Input: part model. Units: mm. Frame: model coordinates. A direction names the side the tool comes from. Round coordinates to 2 decimals unless told otherwise and drop trailing zeros. Loops run counter-clockwise (first coordinate to the right, second up) from the corner with the lowest first, then second, coordinate; pieces in that order, holes last. Notation, with made-up numbers: (85, 37.5) - (129, 37.5) arc R16 ccw to (129, 67.5) - close; hole circle Ø6 at (47.5, 63.5). An arc over 180 degrees is marked (long way). Write each question's results on one line, items separated by ' | '.
from build123d import *

# Parameters (mm, degrees)
EXTRUDE_1_DEPTH     = 15
SKETCH_2_W          = 4
SKETCH_2_H          = 60
EXTRUDE_2_DEPTH     = 10
SKETCH_3_R          = 1.6
CUT_EXTRUDE_1_DEPTH = 6


with BuildPart() as part:
    # ｽｹｯﾁ1 → ﾎﾞｽ - 押し出し1 (new body)
    with BuildSketch(Plane.XY):
        Polygon((-37.26940162, 16.179775281), (-33.26940162, 16.179775281), (-33.26940162, -39.820224719), (-3.26940162, -39.820224719), (-3.26940162, -43.820224719), (-37.26940162, -43.820224719), align=None)
    extrude(amount=EXTRUDE_1_DEPTH)

    # ｽｹｯﾁ2 → ﾎﾞｽ - 押し出し2 (add)
    with BuildSketch(Plane.ZY.offset(37.26940162)):
        with Locations((13, -13.820224719)):
            Rectangle(SKETCH_2_W, SKETCH_2_H)
    extrude(amount=EXTRUDE_2_DEPTH)

    # ｽｹｯﾁ3 → ｶｯﾄ - 押し出し1 (cut)
    with BuildSketch(Plane.XY.offset(15)):
        with Locations((-41.26940162, 7.900067142)):
            Circle(SKETCH_3_R)
        with Locations((-41.26940162, 2.900067142)):
            Circle(SKETCH_3_R)
        with Locations((-41.26940162, -2.099932858)):
            Circle(SKETCH_3_R)
        with Locations((-41.26940162, -7.099932858)):
            Circle(SKETCH_3_R)
        with Locations((-41.26940162, -12.099932858)):
            Circle(SKETCH_3_R)
        with Locations((-41.26940162, -17.099932858)):
            Circle(SKETCH_3_R)
        with Locations((-41.26940162, -22.099932858)):
            Circle(SKETCH_3_R)
        with Locations((-41.26940162, -27.099932858)):
            Circle(SKETCH_3_R)
        with Locations((-41.26940162, -32.099932858)):
            Circle(SKETCH_3_R)
        with Locations((-41.26940162, -37.099932858)):
            Circle(SKETCH_3_R)
        with Locations((-41.26940162, 12.900067142)):
            Circle(SKETCH_3_R)
    extrude(amount=-CUT_EXTRUDE_1_DEPTH, mode=Mode.SUBTRACT)


solid = part.part
1. Line query: line 1 (X direction, y = -22, z = 13); line 2 (Y direction, x = -31.5, z = 13); line 3 (X direction, y = -25, z = 12.25). Output: solid intervals per line, ascending. Write a range as [from, to].
Answer:
line 1: [-47.27, -42.87], [-39.67, -33.27] | line 2: [-43.82, -39.82] | line 3: [-47.27, -33.27]
2. Mould query, pull axis X, two halves, no side actions, for faces 1 (the flat face through (-33.269, -11, 7)), 2 (the cylindrical face through (-39.743, -11.619, 13.028)), 3 (the flat face through (-37.269, -14, 5)). Classes: pulls with the +X half, pulls with the -X half, needs draft (parallel to the pull), parting line crosses it, or undercut.
Answer:
face 1: pulls with the +X half | face 2: undercut | face 3: pulls with the -X half
3. Set-up query: faces 4 (the flat face through (-3.269, -42, 7)), 5 (the flat face through (-18, -39.82, 7)). Return all of +Z, -Z, +X, -X, +Y, -Y with unobstructed straight access to the full face (end or side cutting, diameter ignored); none if empty.
Answer:
face 4: +Z, -Z, +X, +Y, -Y | face 5: +Z, -Z, +X, +Y
4. Section query D-D, the plane x = -28.5. Output: boundary loops of the cut face in (y, z), plus the area to 3 significant figures.
Answer:
outline: (-43.82, 0) - (-39.82, 0) - (-39.82, 15) - (-43.82, 15) - close | area: 60.0 mm^2
5. Section query A-A, the plane y = -8. Output: boundary loops of the cut face in (x, z).
Answer:
outline: (-47.27, 11) - (-42.59, 11) - (-42.59, 15) - (-47.27, 15) - close; (-39.95, 11) - (-37.27, 11) - (-37.27, 0) - (-33.27, 0) - (-33.27, 15) - (-39.95, 15) - close
6. Contact query for flat-ended pins moving along their axis: pin 1 (7.5 mm diameter, centred on y = -24, z = 5, fed in from +X); pin 2 (3.5 mm diameter, centred on x = -41.27, y = -7.1, fed in from -Z); pin 3 (6 mm diameter, centred on x = -11, z = 10.5, fed in from +Y); pin 4 (2.5 mm diameter, centred on x = -41.27, y = -12.1, fed in from -Z). Output: stop coordinate, or through.
Answer:
pin 1: x = -33.27 | pin 2: z = 11 | pin 3: y = -39.82 | pin 4: through
7. Section query C-C, the plane y = -24.5. Output: boundary loops of the cut face in (x, z).
Answer:
outline: (-47.27, 11) - (-37.27, 11) - (-37.27, 0) - (-33.27, 0) - (-33.27, 15) - (-47.27, 15) - close
8. Section query B-B, the plane z = 5.75. Output: boundary loops of the cut face in (x, y).
Answer:
outline: (-37.27, -43.82) - (-3.27, -43.82) - (-3.27, -39.82) - (-33.27, -39.82) - (-33.27, 16.18) - (-37.27, 16.18) - close
